```python
from build123d import *

# Parameters (mm, degrees)
REVOLVE_1_ANGLE      = 180
EXTRUDE_2_DEPTH      = 40
EXTRUDE_2_DEPTH_BACK = 48
SKETCH_3_R           = 1.45
CUT_EXTRUDE_1_DEPTH  = 40


with BuildPart() as part:
    # 草图1 → 旋转1 (revolve)
    with BuildSketch(Plane.XY):
        Polygon((0.445759369, 0), (4.86726431, -2.823603424), (1.86726431, -2.823603424), (-2.554240631, 0), (-2.554240631, 45), (0.445759369, 45), align=None)
    revolve(axis=Axis((25.445759369, 0, 0), (0, 1, 0)), revolution_arc=REVOLVE_1_ANGLE)

    # 草图2 → 凸台-拉伸2 (add, two sides: drawn at the far end of the back side and taken through both)
    with BuildSketch(Plane(origin=(0, 45, 0), x_dir=(1, 0, 0), z_dir=(0, 1, 0)).offset(-EXTRUDE_2_DEPTH_BACK)):
        with BuildLine():
            Line((32.945759369, -30), (32.945759369, -26.97684192))
            ThreePointArc((32.945759369, -26.97684192), (25.445759369, -28), (17.945759369, -26.97684192))
            Line((17.945759369, -26.97684192), (17.945759369, -30))
            Line((17.945759369, -30), (32.945759369, -30))
        make_face()
        with BuildLine():
            Line((32.945759369, -25), (25.445759369, -25))
            Line((25.445759369, -25), (17.945759369, -25))
            Line((17.945759369, -25), (17.945759369, -26.97684192))
            ThreePointArc((17.945759369, -26.97684192), (25.445759369, -28), (32.945759369, -26.97684192))
            Line((32.945759369, -26.97684192), (32.945759369, -25))
        make_face()
    extrude(amount=EXTRUDE_2_DEPTH + EXTRUDE_2_DEPTH_BACK)

    # 草图3 → 切除-拉伸1 (cut)
    with BuildSketch(Plane(origin=(32.945759369, 0, 0), x_dir=(0, 0, -1), z_dir=(1, 0, 0))):
        with Locations((-27.5, 80)):
            Circle(SKETCH_3_R)
    extrude(amount=-CUT_EXTRUDE_1_DEPTH, mode=Mode.SUBTRACT)


solid = part.part
```
Source: CAD feature listing. Evaluate the final solid. Frame: model axes, mm. A direction names the side the tool comes from. Round coordinates to 2 decimals unless told otherwise and drop trailing zeros. Loops run counter-clockwise (first coordinate to the right, second up) from the corner with the lowest first, then second, coordinate; pieces in that order, holes last.
(1) Section query B-B (y = 37.5). Output: boundary loops of the cut face in (x, z).
From the geometry:
outline: (-2.55, 0) - (0.45, 0) arc R25 cw to (50.45, 0) - (53.45, 0) arc R28 ccw to (32.95, 26.98) - (32.95, 30) - (17.95, 30) - (17.95, 26.98) arc R28 ccw to start
(2) Section query C-C (y = 57). Output: boundary loops of the cut face in (x, z), and give its area (3 significant figures).
From the geometry:
outline: (17.95, 25) - (32.95, 25) - (32.95, 30) - (17.95, 30) - close
area: 75.0 mm2
(3) Section query A-A (y = 80). Output: boundary loops of the cut face in (x, z).
From the geometry:
outline: (17.95, 25) - (32.95, 25) - (32.95, 26.05) - (17.95, 26.05) - close; (17.95, 28.95) - (32.95, 28.95) - (32.95, 30) - (17.95, 30) - close
(4) Access query for faces 4 (the flat face through (26, 65, 25)), 5 (the flat face through (27, -2.824, 21)), 6 (the cylindrical face through (24.896, 22.185, 24.994)). Directions: +Z, -Z, +X, -X, +Y, -Y. A direction counts if a zero-diameter tool reaches every point of the face in a straight line with its end or side. Return the directions, or none.
From the geometry:
face 4: -Z, +X, -X, +Y
face 5: -Z, +X, -X, -Y
face 6: -Z, +Y
(5) Pull-direction query (Z, two-part tool) for faces 1 (the flat face through (25, -3, 27)), 2 (the cylindrical face through (25.551, 78.714, 26.831)), 3 (the flat face through (25, 40, 30)); classes: +Z half, -Z half, draft (parallel to the pull), parting line (faces both ways), or undercut.
From the geometry:
face 1: draft
face 2: undercut
face 3: +Z half
(6) Material intervals for probe 1 along Z at (x, y) = (27, 80); probe 2 along Y at (x, z) = (22.5, 27.5); probe 3 along X at (y, z) = (48.5, 25.5), sorted ascending.
From the geometry:
probe 1: z = 25 to 26.05, 28.95 to 30
probe 2: y = -3 to 78.55, 81.45 to 85
probe 3: x = 17.95 to 32.95
(7) Contact query for flat-ended pins moving along their axis: pin 1 Ø1 at (x, z) = (4, 15) entering from +Y; pin 2 Ø0.5 at (x, y) = (22, -1.5) entering from -Z; pin 3 Ø1.5 at (x, z) = (4, 10.5) entering from +Y. Output: stop coordinate, or through.
From the geometry:
pin 1: stops at y = 45
pin 2: stops at z = 21.99
pin 3: stops at y = -0.24
